```python
from build123d import *

# Parameters (mm, degrees)
SKETCH1_W           = 20
SKETCH1_H           = 10
SKETCH1_R           = 1.25
BOSS_EXTRUDE1_DEPTH = 5
SKETCH2_W           = 3
SKETCH2_H           = 10
BOSS_EXTRUDE2_DEPTH = 5
FILLET1_R           = 3


with BuildPart() as part:
    # Sketch1 → Boss-Extrude1 (new body)
    with BuildSketch(Plane(origin=(0, 0, 0), x_dir=(1, 0, 0), z_dir=(0, 1, 0))):
        with Locations((10, 5)):
            Rectangle(SKETCH1_W, SKETCH1_H)
        with Locations((3, 5)):
            Circle(SKETCH1_R, mode=Mode.SUBTRACT)
        with Locations((17, 5)):
            Circle(SKETCH1_R, mode=Mode.SUBTRACT)
    extrude(amount=BOSS_EXTRUDE1_DEPTH)

    # Sketch2 → Boss-Extrude2 (add)
    with BuildSketch(Plane(origin=(0, 5, 0), x_dir=(1, 0, 0), z_dir=(0, 1, 0))):
        with Locations((7.5, 5)):
            Rectangle(SKETCH2_W, SKETCH2_H)
        with Locations((12.5, 5)):
            Rectangle(SKETCH2_W, SKETCH2_H)
    extrude(amount=BOSS_EXTRUDE2_DEPTH)

    # Fillet1
    fillet1_edges = [part.edges().sort_by_distance(p)[0] for p in [
        (0, 2.5, -10),
        (20, 2.5, -10),
        (0, 2.5, 0),
        (20, 2.5, 0),
    ]]
    fillet(fillet1_edges, radius=FILLET1_R)


solid = part.part
```
For this review, take the finished solid that the model builds, in its own axes (mm). A direction names the side the tool comes from. Round coordinates to 2 decimals unless told otherwise and drop trailing zeros. Write each loop counter-clockwise with the first axis right and the second up, starting at its lowest first coordinate (ties: lowest second). Pieces come first, ordered by that corner, then holes. Notation, with made-up numbers: M 27.5,57.25 L 54.5,57.25 A20 cw 54.5,84.25 Z; hole C -12,39 d3. An arc over 180 degrees is marked long. One line per item, written item: value. Start each with the question number.
(1) The part is to be moulded in two halves that separate along Z. For faces 4 (the flat face through (10, 4, -10)), 5 (the flat face through (10, 5, -5)), 6 (the cylindrical face through (16.73, 2.46, -3.78)), say which applies: released by +Z, released by -Z, zero draft, split by the parting line, or undercut.
(2) Machinability: for faces 1 (the flat face through (15.6, 5, -5.1)), 2 (the flat face through (6, 7, -5)), 3 (the flat face through (11, 7, -5)), which of the approach directions +Z, -Z, +X, -X, +Y, -Y give a long, thin tool a straight path to every point of the face, cutting with its end or side? Answer none if there is none.
(3) We need section D-D (y = 1). Give the boundary of the cut face in (x, z).
(4) Wall thickness on line 1 (X direction, y = 3.9, z = -5); line 2 (Z direction, x = 17, y = 1.8); line 3 (X direction, y = 7.75, z = -3.25): over which ranges is each line inside the solid? List them lowest first.
(5) We need section C-C (x = 3.5). Give the boundary of the cut face in (y, z).
(6) Insertion check: pin 1 (2 mm diameter, centred on x = 17.5, y = 5, fed in from -Z); pin 2 (4 mm diameter, centred on y = 7.5, z = -5.5, fed in from -X); pin 3 (1.5 mm diameter, centred on y = 8.5, z = -5, fed in from +X); pin 4 (2 mm diameter, centred on x = 17, z = -5, fed in from -Y). Each pin has a flat end and moves straight along its axis. Give the tip position at first contact, or say it passes through.
(7) We need section B-B (y = 8). Give the boundary of the cut face in (x, z).
(8) We need section A-A (z = -4). Give the boundary of the cut face in (x, y), and give its area (3 significant figures).
Result:
1. face 4: released by -Z
1. face 5: zero draft
1. face 6: undercut
2. face 1: +Z, -Z, +X, +Y
2. face 2: +Z, -Z, -X, +Y
2. face 3: +Z, -Z, +Y
3. outline: M 0,-7 A3 ccw 3,-10 L 17,-10 A3 ccw 20,-7 L 20,-3 A3 ccw 17,0 L 3,0 A3 ccw 0,-3 Z; hole C 3,-5 d2.5; hole C 17,-5 d2.5
4. line 1: 0 to 1.75, 4.25 to 15.75, 18.25 to 20
4. line 2: -10 to -6.25, -3.75 to 0
4. line 3: 6 to 9, 11 to 14
5. outline: M 0,-10 L 5,-10 L 5,-6.15 L 0,-6.15 Z; M 0,-3.85 L 5,-3.85 L 5,0 L 0,0 Z
6. pin 1: z = -10
6. pin 2: x = 6
6. pin 3: x = 14
6. pin 4: through
7. outline: M 6,-10 L 9,-10 L 9,0 L 6,0 Z; M 11,-10 L 14,-10 L 14,0 L 11,0 Z
8. outline: M 0,0 L 2.25,0 L 2.25,5 L 0,5 Z; M 3.75,0 L 16.25,0 L 16.25,5 L 14,5 L 14,10 L 11,10 L 11,5 L 9,5 L 9,10 L 6,10 L 6,5 L 3.75,5 Z; M 17.75,0 L 20,0 L 20,5 L 17.75,5 Z
8. area: 115 mm²
